from build123d import *

# Parameters (mm, degrees)
SKETCH1_W           = 70
SKETCH1_H           = 110
BOSS_EXTRUDE1_DEPTH = 1.25
SKETCH2_W           = 2.5
SKETCH2_H           = 2.5
BOSS_EXTRUDE2_DEPTH = 5
SKETCH3_W           = 60
SKETCH3_H           = 100
CUT_EXTRUDE1_DEPTH  = 0.6


with BuildPart() as part:
    # Sketch1 → Boss-Extrude1 (new body)
    with BuildSketch(Plane(origin=(0, 0, 0), x_dir=(0, 0, -1), z_dir=(1, 0, 0))):
        with Locations((35, 55)):
            Rectangle(SKETCH1_W, SKETCH1_H)
    extrude(amount=BOSS_EXTRUDE1_DEPTH)

    # Sketch2 → Boss-Extrude2 (add)
    with BuildSketch(Plane(origin=(1.25, 0, 0), x_dir=(0, 0, -1), z_dir=(1, 0, 0))):
        with Locations((11.5, 107.5)):
            Rectangle(SKETCH2_W, SKETCH2_H)
        with Locations((11.5, 2.5)):
            Rectangle(SKETCH2_W, SKETCH2_H)
        with Locations((59, 2.5)):
            Rectangle(SKETCH2_W, SKETCH2_H)
    extrude(amount=BOSS_EXTRUDE2_DEPTH)

    # Sketch3 → Cut-Extrude1 (cut)
    with BuildSketch(Plane(origin=(1.25, 0, 0), x_dir=(0, 0, -1), z_dir=(1, 0, 0))):
        with Locations((35, 55)):
            Rectangle(SKETCH3_W, SKETCH3_H)
    extrude(amount=-CUT_EXTRUDE1_DEPTH, mode=Mode.SUBTRACT)


solid = part.part
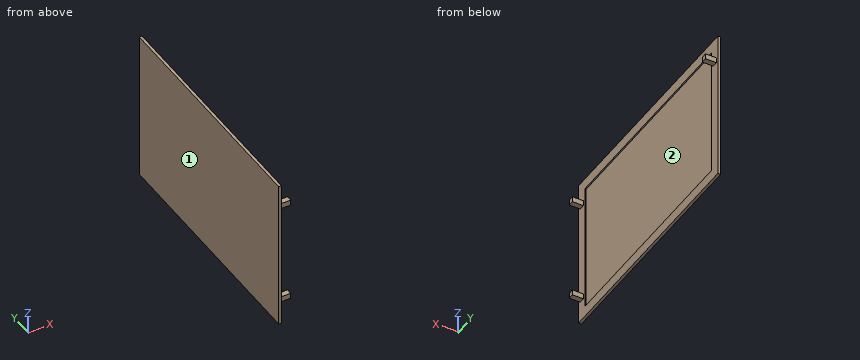
Geometry check sheet. Reference: the model listing, model coordinates, mm. Face numbers are marked on the shaded views. Give positions to 0.01 mm unless a question says otherwise; leave off trailing zeros. Order: outer loops, then holes, each group sorted by start corner. A loop starts at its lowest first (then second) coordinate and runs counter-clockwise, first axis right, second up. Notation, with made-up numbers: M 53.5,60.5 L 83.5,60.5 A18 ccw 83.5,88.5 Z; hole C 39,-29 d9. An arc over 180 degrees is marked long. Use a Markdown table: item, result.
Item 1: Material ranges on line 1 along Y through (x, z) = (5.25, -11.5); line 2 along Y through (x, z) = (0.75, -46); line 3 along X through (y, z) = (74, -49), recorded low to high.
Answers follow:
| item | result |
|---|---|
| line 1 | y = 1.25 to 3.75, 106.25 to 108.75 |
| line 2 | y = 0 to 5, 105 to 110 |
| line 3 | x = 0 to 0.65 |
Item 2: Section check C-C (z = -28.5). Record the cut outline in (x, y), and give its area (3 significant figures).
Answers follow:
| item | result |
|---|---|
| outline | M 0,0 L 1.25,0 L 1.25,5 L 0.65,5 L 0.65,105 L 1.25,105 L 1.25,110 L 0,110 Z |
| area | 77.5 mm2 |
Item 3: Section check A-A (x = 3.5). Record the cut outline in (y, z).
Answers follow:
| item | result |
|---|---|
| outline | M 1.25,-60.25 L 3.75,-60.25 L 3.75,-57.75 L 1.25,-57.75 Z; M 1.25,-12.75 L 3.75,-12.75 L 3.75,-10.25 L 1.25,-10.25 Z; M 106.25,-12.75 L 108.75,-12.75 L 108.75,-10.25 L 106.25,-10.25 Z |
Item 4: Section check B-B (y = 11). Record the cut outline in (x, z).
Answers follow:
| item | result |
|---|---|
| outline | M 0,-70 L 1.25,-70 L 1.25,-65 L 0.65,-65 L 0.65,-5 L 1.25,-5 L 1.25,0 L 0,0 Z |
Item 5: Draft check along Y on the marked faces 1 and 2. Enter one of: +Y half, -Y half, draft (parallel to the pull), parting line (faces both ways), or undercut.
Answers follow:
| item | result |
|---|---|
| face 1 | draft |
| face 2 | undercut |
Item 6: Depth check by flat-ended pin: P1, Ø18, axis at y = 47, z = -24, coming from the +X side; P2, Ø0.8, axis at x = 2.5, z = -12, coming from the -Y side; P3, Ø1.2, axis at x = 5, z = -59, coming from the +Y side. Enter the tip coordinate at first touch or a pass-through.
Answers follow:
| item | result |
|---|---|
| P1 | stops at x = 0.65 |
| P2 | stops at y = 1.25 |
| P3 | stops at y = 3.75 |
